Verification items for the finished model (mm, model axes). A direction names the side the tool comes from. Give positions to 0.01 mm unless a question says otherwise; leave off trailing zeros. Order: outer loops, then holes, each group sorted by start corner. A loop starts at its lowest first (then second) coordinate and runs counter-clockwise, first axis right, second up.
from build123d import *

# Parameters (mm, degrees)
SKETCH068_W      = 3.5
SKETCH068_H      = 3
EXTRUDE058_DEPTH = 1
EXTRUDE057_DEPTH = 28.64


with BuildPart() as extrude058:
    # Sketch068 → Extrude058 (new body, symmetric)
    with BuildSketch(Plane.YZ.offset(311)):
        with Locations((259.75, -21.82)):
            Rectangle(SKETCH068_W, SKETCH068_H)
    extrude(amount=EXTRUDE058_DEPTH, both=True)


with BuildPart() as cut005:
    # Sketch067 → Extrude057 (new body)
    with BuildSketch(Plane(origin=(0, 0, 6.32), x_dir=(1, 0, 0), z_dir=(0, 0, -1))):
        Polygon((321.5, -246), (323, -246), (323, -263), (310, -263), (310, -256), (312, -256), (312, -261.5), (321.5, -261.5), align=None)
    extrude(amount=EXTRUDE057_DEPTH)

    # Cut005: cut Extrude058
    add(extrude058.part, mode=Mode.SUBTRACT)


solid = cut005.part
(1) Section check C-C, the plane y = 260. Enter the section's corners in (x, z).
Solved:
outline: (310, -20.32) - (312, -20.32) - (312, 6.32) - (310, 6.32) - close; (321.5, -22.32) - (323, -22.32) - (323, 6.32) - (321.5, 6.32) - close
(2) Section check A-A, the plane y = 256.75. Enter the section's corners in (x, z).
Solved:
outline: (310, -22.32) - (312, -22.32) - (312, 6.32) - (310, 6.32) - close; (321.5, -22.32) - (323, -22.32) - (323, 6.32) - (321.5, 6.32) - close
(3) Scan lines: line 1 (X direction, y = 258.25, z = 4); line 2 (Y direction, x = 314.5, z = -18.5); line 3 (X direction, y = 247, z = -10.75). Record each from-to range of solid material in increasing order.
Solved:
line 1: x = 310 to 312, 321.5 to 323
line 2: y = 261.5 to 263
line 3: x = 321.5 to 323
(4) Set-up check for faces 4 (the flat face through (322, 257, -22.32)), 5 (the flat face through (311, 260, -20.32)), 6 (the flat face through (322, 246, -8)), 7 (the flat face through (321.5, 254, -8)), 8 (the flat face through (311, 256, -8)): record each of +Z, -Z, +X, -X, +Y, -Y from which the full face is reachable in a straight line by a thin tool's end or side.
Solved:
face 4: -Z, +X, -X, +Y, -Y
face 5: -Z, -X
face 6: +Z, -Z, +X, -X, -Y
face 7: +Z, -Z, -Y
face 8: +Z, -Z, -X, -Y
(5) Section check B-B, the plane z = 0. Enter the section's corners in (x, y), then the cut area to 4 significant figures.
Solved:
outline: (310, 256) - (312, 256) - (312, 261.5) - (321.5, 261.5) - (321.5, 246) - (323, 246) - (323, 263) - (310, 263) - close
area: 53.75 mm2
(6) Go/stop test with flat-tipped pins: pin 1 (1 mm diameter, centred on x = 311, z = -14, fed in from -Y); pin 2 (3.5 mm diameter, centred on x = 316.5, z = -10, fed in from -Y); pin 3 (2 mm diameter, centred on x = 310.5, y = 259.5, fed in from -Z); pin 4 (5 mm diameter, centred on x = 320.5, y = 253.5, fed in from -Z). Record where each tip stops, or that it passes through.
Solved:
pin 1: stops at y = 256
pin 2: stops at y = 261.5
pin 3: stops at z = -20.32
pin 4: stops at z = -22.32
(7) Release check for a two-part mould opening along X. For faces 1 (the flat face through (312, 259, -8)), 2 (the flat face through (322, 258, 6.32)), 3 (the flat face through (323, 254, -8)) record: pulls with the +X half, pulls with the -X half, needs draft (parallel to the pull), parting line crosses it, or undercut.
Solved:
face 1: undercut
face 2: needs draft
face 3: pulls with the +X half
(8) Section check D-D, the plane x = 316.75. Enter the section's corners in (y, z).
Solved:
outline: (261.5, -22.32) - (263, -22.32) - (263, 6.32) - (261.5, 6.32) - close
